Model file for the job. Use its own axes, mm. A direction names the side the tool comes from. Coordinates: 2 decimals unless noted, no trailing zeros. Order: outer loops, then holes, each group sorted by start corner. A loop starts at its lowest first (then second) coordinate and runs counter-clockwise, first axis right, second up. Notation, with made-up numbers: (-20, -4.75) -> (33, -4.75) arc R32 cw to (33, 31.25) -> close; hole circle Ø4 at (78.5, 61.5). An arc over 180 degrees is marked (long way). Use CSV: the item, a comma, the result in double quotes. Start each with the question number.
(1) Pull direction X, two halves, no side cores. Call faces 1 (the cylindrical face through (24.573, 9.633, -150.276)), 2 (the cylindrical face through (3.195, -0.391, -146.57)), 3 (the cylindrical face through (9.56, 0.9, -130.13)): pulls with the +X half, pulls with the -X half, needs draft (parallel to the pull), parting line crosses it, or undercut.
(2) Cut at B-B on x = -7.5. Write the cut outline in (y, z), plus the area to 3 significant figures.
(3) Cut at D-D on x = 15. Write the cut outline in (y, z), plus the area to 3 significant figures.
(4) Pin check, flat tips, straight feed: pin 1 Ø12 at (x, y) = (25, 1) entering from +Z; pin 2 Ø5 at (y, z) = (-7, -143.5) entering from +X; pin 3 Ø11 at (x, y) = (5.5, -6) entering from -Z; pin 4 Ø12 at (x, z) = (5, -143.5) entering from -Y. Stop position of each tip, or through.
(5) Cut at A-A on z = -140. Write the cut outline in (x, y).
(6) Cut at C-C on y = 1. Write the cut outline in (x, z).
(7) Probe L1, parallel to X at y = 11.5, z = -146.5; L2, parallel to X at y = 4.75, z = -140; L3, parallel to Y at x = -10, z = -158. List the from-to ranges inside material, lowest first.
(8) Tool access for faces 4 (the flat face through (13.327, -5, -147)), 5 (the flat face through (-10, 0, -147)), 6 (the flat face through (10, -4, -132.273)), 7 (the flat face through (10, -3, -161.273)), 8 (the flat face through (10, 9, -164.273)): list every direction of +Z, -Z, +X, -X, +Y, -Y with a clear straight run to the whole face (end or side of a thin tool).
Autodesk Inventor part; units mm, degrees
ref_plane "YZ Plane" through (0, 0, 0) normal (1, 0, 0) x (0, 1, 0)
ref_plane "XZ Plane" through (0, 0, 0) normal (0, 1, 0) x (-1, 0, 0)
ref_plane "XY Plane" through (0, 0, 0) normal (0, 0, 1) x (1, 0, 0)
sketch "Schizzo1" plane through (0, 0, 0) normal (0, 1, 0) x (-1, 0, 0)
  line L0 (14.2727, -129.2727) -> (-32.7273, -129.2727)
  line L1 (-32.7273, -129.2727) -> (-32.7273, -164.2727)
  line L2 (-32.7273, -164.2727) -> (14.2727, -164.2727)
  line L3 (14.2727, -164.2727) -> (14.2727, -129.2727)
  line L4 (14.2727, -129.2727) -> (-32.7273, -164.2727) construction
  line L5 (-32.7273, -129.2727) -> (14.2727, -164.2727) construction
  point P0 (0, 0)
  point P1 (-9.2273, -146.7727)
  dimension "d0" = 35
  dimension "d1" = 47
extrude "Estrusione1" add sketch "Schizzo1" along normal blind 19
sketch "Schizzo2" plane through (0, 0, 0) normal (0, -1, 0) x (1, 0, 0)
  line L0 (-14.2727, -129.2727) -> (32.7273, -129.2727)
  line L1 (32.7273, -129.2727) -> (32.7273, -164.2727)
  line L2 (32.7273, -129.2727) -> (32.7273, -164.2727)
  line L3 (32.7273, -146.7727) -> (24.7273, -146.7727)
  line L4 (32.7273, -146.7727) -> (24.7273, -146.7727) construction
  line L5 (24.7273, -146.7727) -> (52.7273, -146.7727) construction
  line L6 (24.7273, -146.7727) -> (24.7273, -153.7727)
  line L7 (24.7273, -146.7727) -> (31.7273, -146.7727) construction
  line L8 (24.7273, -146.7727) -> (24.7273, -139.7727)
  line L9 (24.7273, -146.7727) -> (31.7273, -146.7727) construction
  point P0 (0, 0)
  point P1 (0.7273, -147.0727)
  dimension "d4" = 8
  dimension "d5" = 180
  dimension "d19" = 7
  dimension "d20" = 90
  dimension "d21" = 7
  dimension "d22" = 90
hole "Foro1" at (24.7273, 0, -139.7727) at (24.7273, 0, -153.7727) direction (0, 1, 0) diameter 7 end through all
fillet "Raccordo1" radius 3 1 edges at (9.2273, 19, -129.2727)
fillet "Raccordo2" radius 3 1 edges at (9.2273, 19, -164.2727)
fillet "Raccordo3" radius 3 1 edges at (9.2273, 0, -164.2727)
fillet "Raccordo4" radius 3 1 edges at (9.2273, 0, -129.2727)
sketch "Schizzo3" plane through (0, 19, 0) normal (0, 1, 0) x (1, 0, 0)
  line L0 (32.7273, 146.7727) -> (-6.2727, 146.7727)
  line L1 (32.7273, 146.7727) -> (71.7273, 146.7727) construction
  line L2 (32.7273, 132.2727) -> (32.7273, 161.2727)
  point P0 (0, 0)
  dimension "d23" = 39
  dimension "d24" = 180
hole "Foro2" at (-6.2727, 19, -146.7727) direction (0, -1, 0) diameter 7 end through all
sketch "Schizzo4" plane through (0, 0, 0) normal (0, -1, 0) x (1, 0, 0)
  line L0 (32.7273, -132.2727) -> (32.7273, -161.2727)
  line L1 (8, -215) -> (39.6, -215) construction
  line L2 (13.3273, -161.2727) -> (13.3273, -132.2727)
  line L3 (13.3273, -161.2727) -> (13.3273, -132.2727)
  line L4 (13.3273, -132.2727) -> (3.3273, -132.2727)
  line L5 (3.3273, -132.2727) -> (3.3273, -161.2727)
  line L6 (3.3273, -161.2727) -> (13.3273, -161.2727)
  line L7 (32.7273, -132.2727) -> (-14.2727, -132.2727)
  line L8 (78, -150) -> (86, -150) construction
  line L9 (32.7273, -146.7727) -> (24.7273, -146.7727)
  line L10 (32.7273, -146.7727) -> (40.7273, -146.7727) construction
  line L11 (24.7273, -146.7727) -> (13.3273, -146.7727)
  line L12 (24.7273, -146.7727) -> (36.1273, -146.7727) construction
  point P0 (0, 0)
  dimension "d35" = 29
  dimension "d36" = 10
  dimension "d44" = 8
  dimension "d45" = 180
  dimension "d46" = 11.4
  dimension "d47" = 180
extrude "Estrusione2" add sketch "Schizzo4" along normal blind 10 contours L2 L6 L5 L4
sketch "Schizzo5" plane through (3.3273, 0, -132.2727) normal (0, 0, 1) x (1, 0, 0)
  line L0 (10, 0) -> (10, -10)
  line L1 (10, 0) -> (0, 0)
  line L2 (10, -10) -> (0, 0)
  line L3 (0, -10) -> (10, -10)
  line L4 (0, 0) -> (0, -10)
  line L5 (10, -10) -> (0, -10)
  line L6 (0, -10) -> (0, 0)
  point P0 (-3.3273, 0)
extrude "Estrusione3" cut sketch "Schizzo5" against normal through all contours L3 L4 L2
fillet "Raccordo5" radius 5 1 edges at (3.3273, 0, -146.7727)
properties part number "22_Blocco_Escursione_Braccio" material "PLA(Stampato)(D0,646)"
Outcome:
1,face 1,"undercut"
1,face 2,"pulls with the -X half"
1,face 3,"needs draft"
2,outline,"(0, -161.27) arc R3 ccw to (3, -164.27) -> (16, -164.27) arc R3 ccw to (19, -161.27) -> (19, -150.05) -> (0, -150.05) -> close; (0, -143.49) -> (19, -143.49) -> (19, -132.27) arc R3 ccw to (16, -129.27) -> (3, -129.27) arc R3 ccw to (0, -132.27) -> close"
2,area,"533 mm2"
3,outline,"(0, -161.27) arc R3 ccw to (3, -164.27) -> (16, -164.27) arc R3 ccw to (19, -161.27) -> (19, -132.27) arc R3 ccw to (16, -129.27) -> (3, -129.27) arc R3 ccw to (0, -132.27) -> close"
3,area,"657 mm2"
4,pin 1,"z = -129.27"
4,pin 2,"x = 13.33"
4,pin 3,"z = -161.27"
4,pin 4,"y = -7.67"
5,outline,"(-14.27, 0) -> (1.26, 0) arc R5 cw to (4.79, -1.46) -> (13.33, -10) -> (13.33, 0) -> (21.23, 0) -> (21.23, 19) -> (-14.27, 19) -> close; (28.22, 0) -> (32.73, 0) -> (32.73, 19) -> (28.22, 19) -> close"
6,outline,"(-14.27, -163.51) -> (32.73, -163.51) -> (32.73, -130.04) -> (-14.27, -130.04) -> close; hole circle Ø7 at (-6.27, -146.77); hole circle Ø7 at (24.73, -153.77); hole circle Ø7 at (24.73, -139.77)"
7,L1,"-14.27 to -9.76, -2.78 to 32.73"
7,L2,"-14.27 to 21.23, 28.22 to 32.73"
7,L3,"0 to 19"
8,face 4,"+Z, -Z, +X, -Y"
8,face 5,"+Z, -Z, -X, -Y"
8,face 6,"+Z, +X, -X, -Y"
8,face 7,"-Z, +X, -X, -Y"
8,face 8,"-Z, +X, -X, +Y, -Y"
